from build123d import *

# Parameters (mm, degrees)
F0_R      = 6.35
F1_DEPTH  = 25.4
F2_R      = 25.4
F3_DEPTH  = 38.1
F4_R      = 9.525
F5_DEPTH  = 12.7
F6_R      = 5.08
F7_W      = 38.8537757099
F7_H      = 29.6439938247
F8_DEPTH  = 25.4
F9_DEPTH  = 25.4
F10_DEPTH = 25.4
F11_DEPTH = 56.134


with BuildPart() as f1:
    # F0 (on Right) → F1 (new body)
    with BuildSketch(Plane.YZ):
        Circle(F0_R)
    extrude(amount=F1_DEPTH)

    # F2 (on face) → F3 (join)
    with BuildSketch(Plane.YZ.offset(25.4)):
        Circle(F2_R)
    extrude(amount=F3_DEPTH)

    # F4 (on face) → F5 (cut)
    with BuildSketch(Plane.YZ.offset(63.5)):
        Circle(F4_R)
    extrude(amount=-F5_DEPTH, mode=Mode.SUBTRACT)

    # F6
    f6_edges = [f1.edges().sort_by_distance(p)[0] for p in [
        (63.5, -25.4, 0),
        (63.5, -9.525, 0),
        (25.4, -25.4, 0),
    ]]
    fillet(f6_edges, radius=F6_R)

    # F7 (on Front) → F8 (join)
    with BuildSketch(Plane.XZ):
        with Locations((5.6122131646, 4.7487951815)):
            Rectangle(F7_W, F7_H)
    extrude(amount=F8_DEPTH)

    # F9 (add): a face of the model
    f9_faces = [f1.faces().sort_by_distance(p)[0] for p in [
        (2.9778278266, 0, 6.5599353899),
    ]]
    extrude(f9_faces, amount=F9_DEPTH)

    # F10 (cut): a face of the model
    f10_faces = [f1.faces().sort_by_distance(p)[0] for p in [
        (2.9778278266, 25.4, 6.5599353899),
    ]]
    extrude(f10_faces, amount=-F10_DEPTH, mode=Mode.SUBTRACT)

    # F11 (cut): a face of the model
    f11_faces = [f1.faces().sort_by_distance(p)[0] for p in [
        (5.6122131646, -25.4, 4.7487951815),
    ]]
    extrude(f11_faces, amount=-F11_DEPTH, mode=Mode.SUBTRACT)


solid = f1.part
Can you work these out from the model? Positions are in its coordinate system, mm. A direction names the side the tool comes from. Give positions to 0.01 mm unless a question says otherwise; leave off trailing zeros. Write each loop counter-clockwise with the first axis right and the second up, starting at its lowest first coordinate (ties: lowest second). Pieces come first, ordered by that corner, then holes. Notation, with made-up numbers: M -4.75,-16.75 L 43.25,-16.75 A4 ccw 43.25,-10.75 Z; hole C -22.5,4 d1. An arc over 180 degrees is marked long. Answer in a Markdown table with one row per item. Add a question column.
Item 1: On a 3-axis mill with a long thin cutter (end or side, diameter ignored), from which of +Z, -Z, +X, -X, +Y, -Y can I reach the whole of each face in a straight line? I mean faces 1 (the flat face through (50.8, 0, 0)), 2 (the cylindrical face through (25.22, -1.38, -6.2)), 3 (the flat face through (63.5, -5, 14)). Say none if no direction works.
Item 2: For pin 1 Ø2 at (y, z) = (-17, 11.5) entering from -X; pin 2 Ø20.5 at (y, z) = (7, 2.5) entering from -X; pin 3 Ø3 at (x, y) = (29.5, -15) entering from +Z; pin 4 Ø15 at (y, z) = (2.5, 0) entering from +X, each with a flat end and sliding along its axis, tell me the tip position at first contact or that it passes through.
Item 3: Please list where these lines run through material, in increasing order: L1, parallel to Z at x = 58, y = 0.5; L2, parallel to X at y = -2, z = -16.5; L3, parallel to Z at x = 52.5, y = -4.
Item 4: We'd pull the mould along Y, two halves only. Please class faces 4 (the flat face through (25.039, 0, 0)), 5 (the cylindrical face through (44.254, -5.506, -24.796)), 6 (the cylindrical face through (54.663, -7.559, -5.796)): released by +Y, released by -Y, zero draft, split by the parting line, or undercut.
Item 5: Imagine slicing it at A-A, the plane y = 0. Write out the boundary of the cut face in (x, z) (3 decimals), plus the area to 3 significant figures.
Item 6: Imagine slicing it at C-C, the plane x = 52. Write out the boundary of the cut face in (y, z) (3 decimals).
Evaluation:
| question | item | result |
|---|---|---|
| 1 | face 1 | +X |
| 1 | face 2 | -X |
| 1 | face 3 | +Z, -Z, +X, +Y, -Y |
| 2 | pin 1 | stops at x = 25.4 |
| 2 | pin 2 | stops at x = 25.04 |
| 2 | pin 3 | stops at z = 21.44 |
| 2 | pin 4 | stops at x = 60.56 |
| 3 | L1 | z = -25.4 to -9.51, 9.51 to 25.4 |
| 3 | L2 | x = 25.4 to 63.5 |
| 3 | L3 | z = -25.08 to -8.64, 8.64 to 25.08 |
| 4 | face 4 | zero draft |
| 4 | face 5 | split by the parting line |
| 4 | face 6 | undercut |
| 5 | outline | M 25.039,-6.35 L 25.4,-6.35 L 25.4,-20.32 A5.08 ccw 30.48,-25.4 L 58.42,-25.4 A5.08 ccw 63.5,-20.32 L 63.5,-14.605 A5.08 ccw 58.42,-9.525 L 50.8,-9.525 L 50.8,9.525 L 58.42,9.525 A5.08 ccw 63.5,14.605 L 63.5,20.32 A5.08 ccw 58.42,25.4 L 30.48,25.4 A5.08 ccw 25.4,20.32 L 25.4,6.35 L 25.039,6.35 Z |
| 5 | area | 1,660 mm² |
| 6 | outline | C 0,0 d50.8; hole C 0,0 d19.05 |
